from build123d import *

# Parameters (mm, degrees)
BOSS_EXTRUDE1_DEPTH  = 400
CUT_EXTRUDE1_REACH   = 448.476
SKETCH2_W            = 340
SKETCH2_H            = 81
CUT_EXTRUDE2_REACH   = 448.476
SKETCH4_R            = 3.25
SKETCH5_R            = 2
CUT_EXTRUDE3_DEPTH   = 10
CONVERT_SOLID1_DEPTH = 400


# Read off the part's stored shape, not the designer's step: Convert-Solid1
with BuildPart() as part:
    # Sketch1 → Boss-Extrude1 (new body)
    with BuildSketch(Plane.XY):
        with BuildLine():
            Line((-75, 0), (75, 0))
            ThreePointArc((75, 0), (77.828427125, -1.171572875), (79, -4))
            Line((79, -4), (79, -125))
            Line((79, -125), (77, -125))
            Line((77, -125), (77, -6))
            ThreePointArc((77, -6), (75.828427125, -3.171572875), (73, -2))
            Line((73, -2), (-75, -2))
            Line((-75, -2), (-75, 0))
        make_face()
    extrude(amount=BOSS_EXTRUDE1_DEPTH)

    # Sketch2 → Cut-Extrude1 (cut, up to next)
    with BuildSketch(Plane(origin=(79, 0, 0), x_dir=(0, 0, -1), z_dir=(1, 0, 0)), mode=Mode.PRIVATE) as cut_extrude1_sk1:
        with Locations((-190, -64.5)):
            Rectangle(SKETCH2_W, SKETCH2_H)
    cut_extrude1_tool1 = extrude(cut_extrude1_sk1.sketch, amount=-CUT_EXTRUDE1_REACH, mode=Mode.PRIVATE) & part.part
    add(cut_extrude1_tool1.solids().sort_by_distance((79, -64.5, 190))[0], mode=Mode.SUBTRACT)

    # Sketch4 → Cut-Extrude2 (cut, up to next)
    with BuildSketch(Plane(origin=(79, 0, 0), x_dir=(0, 0, -1), z_dir=(1, 0, 0)), mode=Mode.PRIVATE) as cut_extrude2_sk1:
        with Locations(Location((-385, -14, 0), (0, 0, 90))):
            Circle(SKETCH4_R)
    cut_extrude2_tool1 = extrude(cut_extrude2_sk1.sketch, amount=-CUT_EXTRUDE2_REACH, mode=Mode.PRIVATE) & part.part
    # Sketch4 → Cut-Extrude2 (cut, up to next)
    with BuildSketch(Plane(origin=(79, 0, 0), x_dir=(0, 0, -1), z_dir=(1, 0, 0)), mode=Mode.PRIVATE) as cut_extrude2_sk2:
        with Locations(Location((-385, -115, 0), (0, 0, 90))):
            Circle(SKETCH4_R)
    cut_extrude2_tool2 = extrude(cut_extrude2_sk2.sketch, amount=-CUT_EXTRUDE2_REACH, mode=Mode.PRIVATE) & part.part
    add(cut_extrude2_tool1.solids().sort_by_distance((79, -14, 385))[0], mode=Mode.SUBTRACT)
    add(cut_extrude2_tool2.solids().sort_by_distance((79, -115, 385))[0], mode=Mode.SUBTRACT)

    # Sketch5 → Cut-Extrude3 (cut)
    with BuildSketch(Plane(origin=(79, 0, 0), x_dir=(0, 0, -1), z_dir=(1, 0, 0))):
        with Locations(Location((-50, -115, 0), (0, 0, 90))):
            Circle(SKETCH5_R)
        with Locations(Location((-200, -115, 0), (0, 0, 90))):
            Circle(SKETCH5_R)
        with Locations(Location((-350, -115, 0), (0, 0, 90))):
            Circle(SKETCH5_R)
        with Locations(Location((-350, -14, 0), (0, 0, 90))):
            Circle(SKETCH5_R)
        with Locations(Location((-200, -14, 0), (0, 0, 90))):
            Circle(SKETCH5_R)
        with Locations(Location((-50, -14, 0), (0, 0, 90))):
            Circle(SKETCH5_R)
    extrude(amount=-CUT_EXTRUDE3_DEPTH, mode=Mode.SUBTRACT)

    # Convert-Solid1 outline → Convert-Solid1 (cut)
    with BuildSketch(Plane.XY):
        with BuildLine():
            ThreePointArc((77, -4), (76.414213562, -2.585786438), (75, -2))
            Line((75, -2), (73, -2))
            ThreePointArc((73, -2), (75.828427125, -3.171572875), (77, -6))
            Line((77, -6), (77, -4))
        make_face()
    extrude(amount=CONVERT_SOLID1_DEPTH, mode=Mode.SUBTRACT)


solid = part.part
Geometry check sheet. Reference: the model listing, model coordinates, mm. A direction names the side the tool comes from. Give positions to 0.01 mm unless a question says otherwise; leave off trailing zeros. Loops run counter-clockwise (first coordinate to the right, second up) from the corner with the lowest first, then second, coordinate; pieces in that order, holes last. Notation, with made-up numbers: M 88.25,-19 L 136.25,-19 A29 ccw 136.25,12 Z; hole C -19,76.25 d11. An arc over 180 degrees is marked long. Answer as a JSON object with one key per item and string values. Group by question number.
Item 1: Material ranges on L1, parallel to Z at x = 78, y = -115; L2, parallel to Y at x = 77.75, z = 200; L3, parallel to Y at x = 77.85, z = 200, recorded low to high.
Item 2: Access from +Z, -Z, +X, -X, +Y, -Y to the whole of each face (thin tool, end or side, straight path). Record for faces 1 (the flat face through (1, -2, 197)), 2 (the flat face through (-1, 0, 197)).
Item 3: Sectioned sample at A-A on y = -38. Record the boundary of the cut face in (x, z), plus the area to 3 significant figures.
Item 4: Gauge pin test, flat ends, axial feed: pin 1 (5 mm diameter, centred on x = 50.5, z = 340, fed in from -Y); pin 2 (2 mm diameter, centred on x = 78, z = 243.5, fed in from +Y); pin 3 (4.5 mm diameter, centred on y = -14, z = 350, fed in from -X). Record the tip position at first contact, or that the pin passes through.
Item 5: Sectioned sample at B-B on z = 103.5. Record the boundary of the cut face in (x, y).
Item 6: Sectioned sample at C-C on x = 64. Record the boundary of the cut face in (y, z).
Findings below:
{
 "1": {"L1": "0 to 48, 52 to 198, 202 to 348, 352 to 381.75, 388.25 to 400", "L2": "-125 to -117, -113 to -105, -24 to -16, -12 to -1.1", "L3": "-125 to -117, -113 to -105, -24 to -16, -12 to -1.19"},
 "2": {"face 1": "+Z, -Z, -X, -Y", "face 2": "+Z, -Z, +X, -X, +Y"},
 "3": {"outline": "M 77,0 L 79,0 L 79,20 L 77,20 Z; M 77,360 L 79,360 L 79,400 L 77,400 Z", "area": "120 mm2"},
 "4": {"pin 1": "y = -2", "pin 2": "y = -0.54", "pin 3": "x = 77"},
 "5": {"outline": "M -75,-2 L 75,-2 A2 cw 77,-4 L 77,-24 L 79,-24 L 79,-4 A4 ccw 75,0 L -75,0 Z; M 77,-125 L 79,-125 L 79,-105 L 77,-105 Z"},
 "6": {"outline": "M -2,0 L 0,0 L 0,400 L -2,400 Z"}
}
